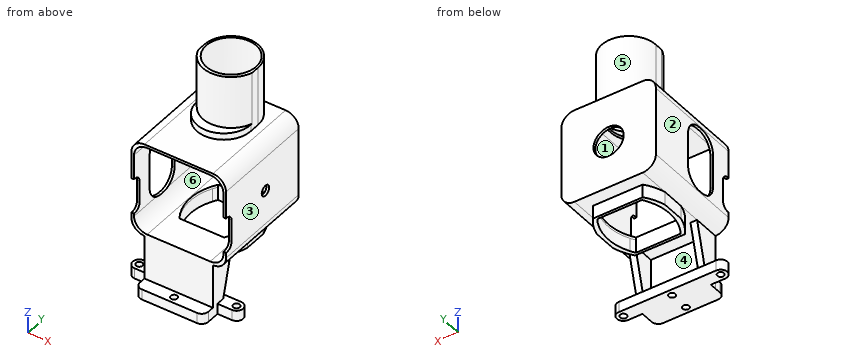
from build123d import *

# Parameters (mm, degrees)
F0_R      = 11.5
F1_DEPTH  = 2
F3_DEPTH  = 77
F5_DEPTH  = 3
F7_DEPTH  = 3
F9_DEPTH  = 5
F11_DEPTH = 3
F12_R     = 19
F13_DEPTH = 8
F14_R     = 19
F15_DEPTH = 40
F16_W     = 52
F16_H     = 3
F17_DEPTH = 38.5
F19_DEPTH = 3
F21_DEPTH = 10
F22_W     = 3
F22_H     = 38.5
F23_DEPTH = 5
F25_R     = 2.5
F25_W     = 47
F25_H     = 2
F26_DEPTH = 5
F27_DEPTH = 1
F29_DEPTH = 75
F30_DEPTH = 2
F24_W     = 3
F24_H     = 38.5
F31_DEPTH = 5
F32_R     = 4
F33_DEPTH = 3


with BuildPart() as f1:
    # F0 (on Front) → F1 (new body)
    with BuildSketch(Plane.XZ):
        with BuildLine():
            Line((26, 36), (-26, 36))
            ThreePointArc((-26, 36), (-33.0710678119, 33.0710678119), (-36, 26))
            Line((-36, 26), (-36, -26))
            ThreePointArc((-36, -26), (-33.0710678119, -33.0710678119), (-26, -36))
            Line((-26, -36), (26, -36))
            ThreePointArc((26, -36), (33.0710678119, -33.0710678119), (36, -26))
            Line((36, -26), (36, 26))
            ThreePointArc((36, 26), (33.0710678119, 33.0710678119), (26, 36))
        make_face()
        with BuildLine():
            Line((24, -34), (-24, -34))
            ThreePointArc((-24, -34), (-31.0710678119, -31.0710678119), (-34, -24))
            Line((-34, -24), (-34, 24))
            ThreePointArc((-34, 24), (-31.0710678119, 31.0710678119), (-24, 34))
            Line((-24, 34), (24, 34))
            ThreePointArc((24, 34), (31.0710678119, 31.0710678119), (34, 24))
            Line((34, 24), (34, -24))
            ThreePointArc((34, -24), (31.0710678119, -31.0710678119), (24, -34))
        make_face(mode=Mode.SUBTRACT)
        with BuildLine():
            ThreePointArc((-34, -24), (-31.0710678119, -31.0710678119), (-24, -34))
            Line((-24, -34), (24, -34))
            ThreePointArc((24, -34), (31.0710678119, -31.0710678119), (34, -24))
            Line((34, -24), (34, 24))
            ThreePointArc((34, 24), (31.0710678119, 31.0710678119), (24, 34))
            Line((24, 34), (-24, 34))
            ThreePointArc((-24, 34), (-31.0710678119, 31.0710678119), (-34, 24))
            Line((-34, 24), (-34, -24))
        make_face()
        Circle(F0_R, mode=Mode.SUBTRACT)
    extrude(amount=F1_DEPTH)

    # F2 (on face) → F3 (join)
    with BuildSketch(Plane.XZ.offset(2)):
        with BuildLine():
            Line((26, 36), (-26, 36))
            ThreePointArc((-26, 36), (-33.0710678119, 33.0710678119), (-36, 26))
            Line((-36, 26), (-36, -26))
            ThreePointArc((-36, -26), (-33.0710678119, -33.0710678119), (-26, -36))
            Line((-26, -36), (26, -36))
            ThreePointArc((26, -36), (33.0710678119, -33.0710678119), (36, -26))
            Line((36, -26), (36, 26))
            ThreePointArc((36, 26), (33.0710678119, 33.0710678119), (26, 36))
        make_face()
        with BuildLine():
            Line((24, -34), (-24, -34))
            ThreePointArc((-24, -34), (-31.0710678119, -31.0710678119), (-34, -24))
            Line((-34, -24), (-34, 24))
            ThreePointArc((-34, 24), (-31.0710678119, 31.0710678119), (-24, 34))
            Line((-24, 34), (24, 34))
            ThreePointArc((24, 34), (31.0710678119, 31.0710678119), (34, 24))
            Line((34, 24), (34, -24))
            ThreePointArc((34, -24), (31.0710678119, -31.0710678119), (24, -34))
        make_face(mode=Mode.SUBTRACT)
    extrude(amount=F3_DEPTH)

    # F4 (on face) → F5 (cut)
    with BuildSketch(Plane(origin=(-36, 0, 0), x_dir=(0, -1, 0), z_dir=(-1, 0, 0))):
        with BuildLine():
            ThreePointArc((62, 13), (58.4852813742, 21.4852813742), (50, 25))
            Line((50, 25), (47, 25))
            ThreePointArc((47, 25), (38.5147186258, 21.4852813742), (35, 13))
            Line((35, 13), (35, -13))
            ThreePointArc((35, -13), (38.5147186258, -21.4852813742), (47, -25))
            Line((47, -25), (50, -25))
            ThreePointArc((50, -25), (58.4852813742, -21.4852813742), (62, -13))
            Line((62, -13), (62, 13))
        make_face()
    extrude(amount=-F5_DEPTH, mode=Mode.SUBTRACT)

    # F6 (on face) → F7 (cut)
    with BuildSketch(Plane.XY.offset(36)):
        with BuildLine():
            Line((19, -30), (19, -22))
            ThreePointArc((19, -22), (0, -3), (-19, -22))
            Line((-19, -22), (-19, -30))
            ThreePointArc((-19, -30), (0, -49), (19, -30))
        make_face()
    extrude(amount=-F7_DEPTH, mode=Mode.SUBTRACT)

    # F8 (on face) → F9 (join)
    with BuildSketch(Plane.XY.offset(36)):
        with BuildLine():
            Line((-20.5, -22), (-20.5, -30))
            ThreePointArc((-20.5, -30), (0, -50.5), (20.5, -30))
            Line((20.5, -30), (20.5, -22))
            ThreePointArc((20.5, -22), (0, -1.5), (-20.5, -22))
        make_face()
        with BuildLine():
            ThreePointArc((-19, -22), (0, -3), (19, -22))
            Line((19, -22), (19, -22.3025978408))
            Line((19, -22.3025978408), (19, -29.6974021592))
            Line((19, -29.6974021592), (19, -30))
            ThreePointArc((19, -30), (0, -49), (-19, -30))
            Line((-19, -30), (-19, -22))
        make_face(mode=Mode.SUBTRACT)
        with BuildLine():
            Line((19, -22.3025978408), (19, -22))
            ThreePointArc((19, -22), (0, -3), (-19, -22))
            Line((-19, -22), (-19, -30))
            ThreePointArc((-19, -30), (0, -49), (19, -30))
            Line((19, -30), (19, -29.6974021592))
            Line((19, -29.6974021592), (19, -22.3025978408))
        make_face()
    extrude(amount=F9_DEPTH)

    # F10 (on face) → F11 (join)
    with BuildSketch(Plane.XY.offset(36)):
        with BuildLine():
            Line((20.5, -30), (20.5, -22))
            ThreePointArc((20.5, -22), (0, -1.5), (-20.5, -22))
            Line((-20.5, -22), (-20.5, -30))
            ThreePointArc((-20.5, -30), (0, -50.5), (20.5, -30))
        make_face()
    extrude(amount=F11_DEPTH)

    # F12 (on face) → F13 (cut)
    with BuildSketch(Plane.XY.offset(41)):
        with Locations((0, -22)):
            Circle(F12_R)
    extrude(amount=-F13_DEPTH, mode=Mode.SUBTRACT)

    # F14 (on face) → F15 (join)
    with BuildSketch(Plane.XY.offset(41)):
        with BuildLine():
            Line((-20.5, -22), (-20.5, -28.4807406984))
            ThreePointArc((-20.5, -28.4807406984), (0, -43.5), (20.5, -28.4807406984))
            Line((20.5, -28.4807406984), (20.5, -22))
            ThreePointArc((20.5, -22), (0, -1.5), (-20.5, -22))
        make_face()
        with Locations((0, -22)):
            Circle(F14_R, mode=Mode.SUBTRACT)
    extrude(amount=F15_DEPTH)

    # F16 (on face) → F17 (join)
    with BuildSketch(Plane(origin=(0, 0, -36), x_dir=(1, 0, 0), z_dir=(0, 0, -1))):
        with Locations((0, 77.5)):
            Rectangle(F16_W, F16_H)
    extrude(amount=F17_DEPTH)

    # F18 (on face) → F19 (cut)
    with BuildSketch(Plane(origin=(0, 0, -36), x_dir=(1, 0, 0), z_dir=(0, 0, -1))):
        with BuildLine():
            Line((-17, 12), (17, 12))
            ThreePointArc((17, 12), (23.3298247558, 33), (17, 54))
            Line((17, 54), (-17, 54))
            ThreePointArc((-17, 54), (-23.3298247558, 33), (-17, 12))
        make_face()
    extrude(amount=-F19_DEPTH, mode=Mode.SUBTRACT)

    # F20 (on face) → F21 (join)
    with BuildSketch(Plane(origin=(0, 0, -36), x_dir=(1, 0, 0), z_dir=(0, 0, -1))):
        with BuildLine():
            ThreePointArc((19, 50.6158820109), (23.3298247558, 33), (19, 15.3841179891))
            Line((19, 15.3841179891), (19, 10))
            ThreePointArc((19, 10), (23.2866263695, 16.8090036252), (26, 24.3836521016))
            Line((26, 24.3836521016), (26, 41.6163478984))
            ThreePointArc((26, 41.6163478984), (23.2866263695, 49.1909963748), (19, 56))
            Line((19, 56), (19, 50.6158820109))
        make_face()
        with BuildLine():
            Line((-19, 56), (-19, 50.6158820109))
            ThreePointArc((-19, 50.6158820109), (-18.0437883513, 52.3338197434), (-17, 54))
            Line((-17, 54), (17, 54))
            ThreePointArc((17, 54), (18.0437883513, 52.3338197434), (19, 50.6158820109))
            Line((19, 50.6158820109), (19, 56))
            Line((19, 56), (-19, 56))
        make_face()
        with BuildLine():
            Line((-19, 10), (-19, 15.3841179891))
            ThreePointArc((-19, 15.3841179891), (-23.3298247558, 33), (-19, 50.6158820109))
            Line((-19, 50.6158820109), (-19, 56))
            ThreePointArc((-19, 56), (-23.2866263695, 49.1909963748), (-26, 41.6163478984))
            Line((-26, 41.6163478984), (-26, 24.3836521016))
            ThreePointArc((-26, 24.3836521016), (-23.2866263695, 16.8090036252), (-19, 10))
        make_face()
        with BuildLine():
            Line((17, 12), (-17, 12))
            ThreePointArc((-17, 12), (-18.0437883513, 13.6661802566), (-19, 15.3841179891))
            Line((-19, 15.3841179891), (-19, 10))
            Line((-19, 10), (19, 10))
            Line((19, 10), (19, 15.3841179891))
            ThreePointArc((19, 15.3841179891), (18.0437883513, 13.6661802566), (17, 12))
        make_face()
    extrude(amount=F21_DEPTH)

    # F22 (on face) → F23 (join)
    with BuildSketch(Plane.YZ.offset(26)):
        Polygon((-76, -36), (-76, -74.5), (-69, -74.5), (-59, -36), align=None)
        with Locations((-77.5, -55.25)):
            Rectangle(F22_W, F22_H)
    extrude(amount=-F23_DEPTH)

    # F25 (on face) → F26 (join)
    with BuildSketch(Plane(origin=(0, 0, -74.5), x_dir=(1, 0, 0), z_dir=(0, 0, -1))):
        with BuildLine():
            Line((37, 74), (26, 74))
            Line((26, 74), (21, 74))
            Line((21, 74), (-26, 74))
            Line((-26, 74), (-37, 74))
            ThreePointArc((-37, 74), (-42, 69), (-37, 64))
            Line((-37, 64), (37, 64))
            ThreePointArc((37, 64), (42, 69), (37, 74))
        make_face()
        with Locations((-37, 69)):
            Circle(F25_R, mode=Mode.SUBTRACT)
        with Locations((0, 69)):
            Circle(F25_R, mode=Mode.SUBTRACT)
        with Locations((37, 69)):
            Circle(F25_R, mode=Mode.SUBTRACT)
        Polygon((26, 79), (-26, 79), (-26, 76), (21, 76), (21, 74), (26, 74), align=None)
        with Locations((-2.5, 75)):
            Rectangle(F25_W, F25_H)
        with BuildLine():
            Line((-26.0336585343, 79), (-26, 79))
            Line((-26, 79), (26, 79))
            Line((26, 79), (26, 84))
            ThreePointArc((26, 84), (24.5355339059, 87.5355339059), (21, 89))
            Line((21, 89), (-21.0336585343, 89))
            ThreePointArc((-21.0336585343, 89), (-24.5691924402, 87.5355339059), (-26.0336585343, 84))
            Line((-26.0336585343, 84), (-26.0336585343, 79))
        make_face()
        with Locations((0, 84)):
            Circle(F25_R, mode=Mode.SUBTRACT)
    extrude(amount=-F26_DEPTH)

    # F27 (add): faces of the model
    f27_faces = [f1.faces().sort_by_distance(p)[0] for p in [
        (23.5, -77.5, -74.5),
        (-2.5, -77.5, -74.5),
        (23.5, -72.5, -74.5),
        (-26.0168292671, -79.5298586246, -74.5),
        (-41.1514718626, -69, -74.5),
    ]]
    extrude(f27_faces, amount=F27_DEPTH)

    # F28 (on face) → F29 (cut)
    with BuildSketch(Plane.YZ.offset(36)):
        with BuildLine():
            Line((-78, 5), (-79, 5))
            Line((-79, 5), (-79, -22))
            Line((-79, -22), (-78, -22))
            ThreePointArc((-78, -22), (-74.4644660941, -20.5355339059), (-73, -17))
            Line((-73, -17), (-73, 0))
            ThreePointArc((-73, 0), (-74.4644660941, 3.5355339059), (-78, 5))
        make_face()
    extrude(amount=-F29_DEPTH, mode=Mode.SUBTRACT)

    # F30 (add): a face of the model
    f30_faces = [f1.faces().sort_by_distance(p)[0] for p in [
        (-0.0056811519, -75.1326620312, -75.5),
    ]]
    extrude(f30_faces, amount=F30_DEPTH)

    # F24 (on face) → F31 (join)
    with BuildSketch(Plane(origin=(-26, 0, 0), x_dir=(0, -1, 0), z_dir=(-1, 0, 0))):
        with Locations((77.5, -55.25)):
            Rectangle(F24_W, F24_H)
        Polygon((69, -74.5), (76, -74.5), (76, -36), (59, -36), align=None)
    extrude(amount=-F31_DEPTH)

    # F32 (on face) → F33 (cut)
    with BuildSketch(Plane.YZ.offset(36)):
        with Locations((-36.2, 0)):
            Circle(F32_R)
    extrude(amount=-F33_DEPTH, mode=Mode.SUBTRACT)


solid = f1.part
Could you check a few things on this model? Use its own coordinates, in mm. Face numbers are marked on the shaded views. A direction names the side the tool comes from. Coordinates: 2 decimals unless noted, no trailing zeros. Order: outer loops, then holes, each group sorted by start corner. A loop starts at its lowest first (then second) coordinate and runs counter-clockwise, first axis right, second up. Notation, with made-up numbers: (33.5, -16) -> (80.5, -16) arc R24 ccw to (80.5, 22) -> close; hole circle Ø2 at (-28.5, 30). An arc over 180 degrees is marked (long way). One line per question, with ' | ' between items.
Q1. Imagine slicing it at C-C on z = 64. Please give me the cut outline in (x, y).
Return value:
outline: (-20.5, -28.48) arc R21.5 ccw to (20.5, -28.48) -> (20.5, -22) arc R20.5 ccw to (-20.5, -22) -> close; hole circle Ø38 at (0, -22)
Q2. Imagine slicing it at A-A on z = 16. Please give me the cut outline in (x, y), and give its area (3 significant figures).
Return value:
outline: (-36, -79) -> (-34, -79) -> (-34, -61.62) -> (-36, -61.62) -> close; (-36, -35.38) -> (-34, -35.38) -> (-34, -2) -> (34, -2) -> (34, -79) -> (36, -79) -> (36, 0) -> (-36, 0) -> close | area: 400 mm²
Q3. Thinking about a two-plate mould opening in X: for the marked faces 1, 2 and 3, which applies, pulls with the +X half, pulls with the -X half, needs draft (parallel to the pull), parting line crosses it, or undercut?
Return value:
face 1: undercut | face 2: pulls with the -X half | face 3: pulls with the +X half
Q4. On a 3-axis mill with a long thin cutter (end or side, diameter ignored), from which of +Z, -Z, +X, -X, +Y, -Y can I reach the whole of each face in a straight line? I mean the marked faces 4, 5 and 6. Say none if no direction works.
Return value:
face 4: none | face 5: +Z, +Y | face 6: -Y
Q5. Imagine slicing it at B-B on x = 0. State how many separate pieces and enclosed holes the cut face has, and give its area (4 significant figures).
Return value:
separate pieces: 6 | enclosed holes: 0 | area: 705.5 mm²
Q6. I'm going to push flat-ended pins straight in: P1, Ø2.5, axis at x = -3.5, z = -73.5, coming from the +Y side; P2, Ø10, axis at y = -65.5, z = 40, coming from the +X side; P3, Ø10, axis at y = -14.5, z = -36.5, coming from the -X side. Where does each tip first touch, or does it pass through?
Return value:
P1: y = -64 | P2: x = 30.36 | P3: x = -34.35
Q7. Imagine slicing it at D-D on z = -60.5. Please give me the cut outline in (x, y).
Return value:
outline: (-26, -79) -> (26, -79) -> (26, -65.36) -> (21, -65.36) -> (21, -76) -> (-21, -76) -> (-21, -65.36) -> (-26, -65.36) -> close
Q8. If I drill on L1, parallel to Z at x = -4, y = -65; L2, parallel to Y at x = 0, z = -73.5; L3, parallel to X at y = -69, z = -72, over which ranges is the centre line in solid material (lowest first)?
Return value:
L1: -77.5 to -69.5, -36 to -34, 34 to 36 | L2: -89 to -86.5, -81.5 to -71.5, -66.5 to -64 | L3: -42 to -39.5, -34.5 to -2.5, 2.5 to 34.5, 39.5 to 42
